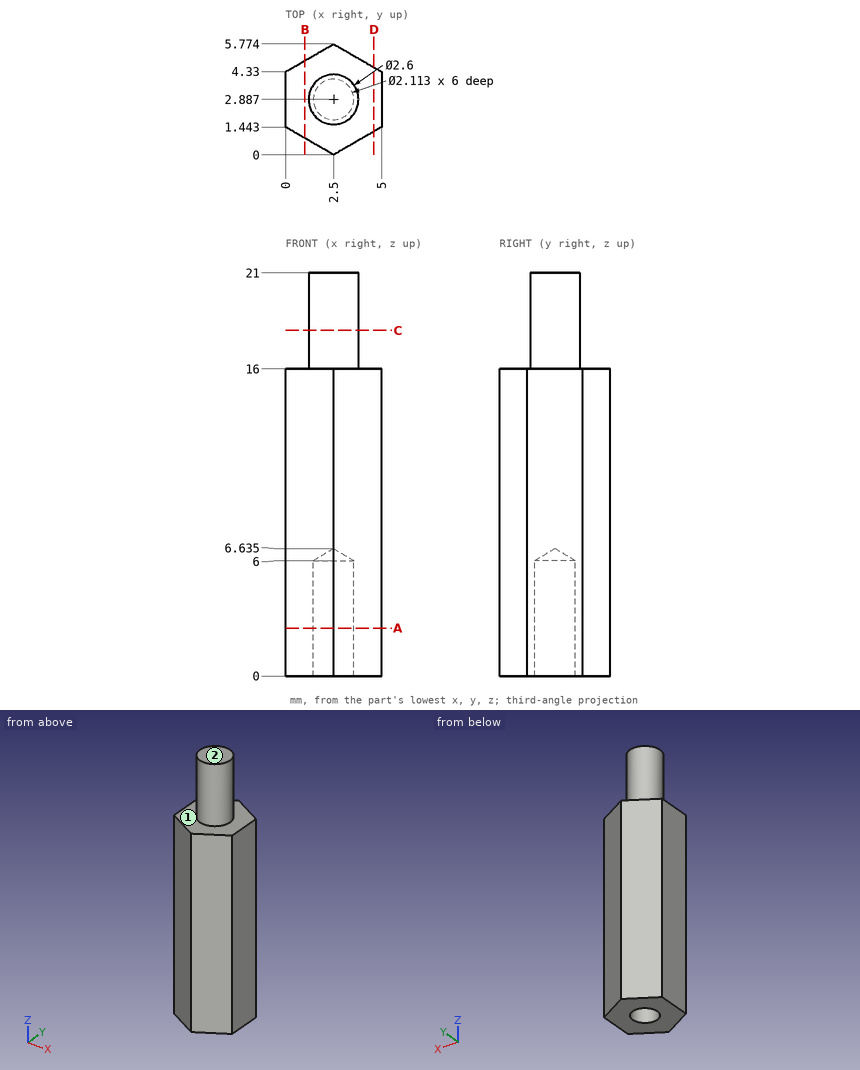
The drawing under review shows one solid part. Ordinate dimensions are in mm from its lowest x, y, z. A direction names the side the tool comes from. Give positions to 0.01 mm unless a question says otherwise; leave off trailing zeros. Write each loop counter-clockwise with the first axis right and the second up, starting at its lowest first coordinate (ties: lowest second). Pieces come first, ordered by that corner, then holes. Notation, with made-up numbers: M 79,-32.5 L 85,-32.5 A16 cw 85,-1.5 Z; hole C -13,-26 d11. An arc over 180 degrees is marked long. Write each question's results on one line, items separated by ' | '. Start each with the question number.
1. For probe 1 along Z at (x, y) = (1.05, 4.9); probe 2 along Y at (x, z) = (1.8, 3) (1 decimal); probe 3 along X at (y, z) = (3.55, 1), list the stretches that pass through material, from the lowest coordinate up. Write a range as [from, to].
2. Insertion check: pin 1 Ø1.7 at (x, y) = (2.5, 2.89) entering from -Z. The pin has a flat end and moves straight along its axis. Give the tip position at first contact, or say it passes through.
3. We need section C-C (z = 18). Write out the cut boundary in (x, y).
4. We need section A-A (z = 2.5). Write out the cut boundary in (x, y).
5. We need section B-B (x = 1). Write out the cut boundary in (y, z).
6. We need section D-D (x = 4.6). Write out the cut boundary in (y, z).
7. For the marked faces 1 and 2, list the 3-axis set-ups (+Z, -Z, +X, -X, +Y, -Y) from which the entire face can be reached by the end or side of a thin tool; tool diameter is ignored.
Results found:
1) probe 1: z = [0, 16] | probe 2: y = [0.4, 2.1], [3.7, 5.4] | probe 3: x = [0, 1.68], [3.32, 5]
2) pin 1: stops at z = 6.12
3) outline: C 2.5,2.89 d2.6
4) outline: M 0,1.44 L 2.5,0 L 5,1.44 L 5,4.33 L 2.5,5.77 L 0,4.33 Z; hole C 2.5,2.89 d2.11
5) outline: M 0.87,0 L 4.91,0 L 4.91,16 L 0.87,16 Z
6) outline: M 1.21,0 L 4.56,0 L 4.56,16 L 1.21,16 Z
7) face 1: +Z | face 2: +Z, +X, -X, +Y, -Y
